Geometry: final body of the model. Coordinates: model frame, mm. A direction names the side the tool comes from. Give positions to 0.01 mm unless a question says otherwise; leave off trailing zeros. Write each loop counter-clockwise with the first axis right and the second up, starting at its lowest first coordinate (ties: lowest second). Pieces come first, ordered by that corner, then holes. Notation, with made-up numbers: M 67.25,31.25 L 119.25,31.25 A20 ccw 119.25,70.25 Z; hole C -39,55.25 d2. An arc over 180 degrees is marked long. One line per question, with ' | ' between items.
from build123d import *

# Parameters (mm, degrees)
BOX003_W               = 4.5
BOX003_H               = 5
BOX003_DEPTH           = 6
BOX003_PLACEMENT_ANGLE = 315
FILLET004_R            = 2.24
BOX002_W               = 19.2
BOX002_H               = 16.5
BOX002_DEPTH           = 6
FILLET005_R            = 2
BOX006_W               = 4.5
BOX006_H               = 5
BOX006_DEPTH           = 6
BOX006_PLACEMENT_ANGLE = 315
FILLET006_R            = 2.24
CYLINDER_R             = 9.75
CYLINDER_DEPTH         = 6
FILLET007_1_R          = 2
FILLET007_2_R          = 1


with BuildPart() as fillet004:
    # Box003 → Box003 (new body)
    with BuildSketch(Plane.XY):
        with Locations((2.25, 2.5)):
            Rectangle(BOX003_W, BOX003_H)
    extrude(amount=BOX003_DEPTH)


with BuildPart() as fillet004_1:
    # Box003 placement: moved
    add(fillet004.part.moved(Location((13.42, 28.5, 0))).rotate(Axis((13.42, 28.5, 0), (0, 0, 1)), BOX003_PLACEMENT_ANGLE))

    # Fillet004
    fillet004_edges = [fillet004_1.edges().sort_by_distance(p)[0] for p in [
        (16.955534, 32.035534, 3),
        (20.137514, 28.853553, 3),
    ]]
    fillet(fillet004_edges, radius=FILLET004_R)


with BuildPart() as fillet005:
    # Box002 → Box002 (new body)
    with BuildSketch(Plane.XY):
        with Locations((9.6, 8.25)):
            Rectangle(BOX002_W, BOX002_H)
    extrude(amount=BOX002_DEPTH)

    # Fillet005
    fillet005_edges = [fillet005.edges().sort_by_distance(p)[0] for p in [
        (0, 0, 3),
        (0, 16.5, 3),
        (19.2, 0, 3),
        (19.2, 16.5, 3),
    ]]
    fillet(fillet005_edges, radius=FILLET005_R)


with BuildPart() as fillet006:
    # Box006 → Box006 (new body)
    with BuildSketch(Plane.XY):
        with Locations((2.25, 2.5)):
            Rectangle(BOX006_W, BOX006_H)
    extrude(amount=BOX006_DEPTH)


with BuildPart() as fillet006_1:
    # Box006 placement: moved
    add(fillet006.part.moved(Location((2.6, 25.3, 0))).rotate(Axis((2.6, 25.3, 0), (0, 0, -1)), BOX006_PLACEMENT_ANGLE))

    # Fillet006
    fillet006_edges = [fillet006_1.edges().sort_by_distance(p)[0] for p in [
        (-0.935534, 28.835534, 3),
        (2.246447, 32.017514, 3),
    ]]
    fillet(fillet006_edges, radius=FILLET006_R)


with BuildPart() as fillet007:
    # Cylinder → Cylinder (new body)
    with BuildSketch(Plane(origin=(9.6, 21.3, 0), x_dir=(1, 0, 0), z_dir=(0, 0, 1))):
        Circle(CYLINDER_R)
    extrude(amount=CYLINDER_DEPTH)

    # Fusion025: union Fillet004, Fillet005, Fillet006
    add(fillet004_1.part)
    add(fillet005.part)
    add(fillet006_1.part)

    # Fillet007 1
    fillet007_1_edges = [fillet007.edges().sort_by_distance(p)[0] for p in [
        (4.596011, 29.66795, 3),
        (14.593947, 29.673947, 3),
        (17.822898, 26.538937, 3),
        (1.370866, 26.529134, 3),
    ]]
    fillet(fillet007_1_edges, radius=FILLET007_1_R)

    # Fillet007 2
    fillet007_2_edges = [fillet007.edges().sort_by_distance(p)[0] for p in [
        (1.207976, 16.336491, 3),
        (17.992024, 16.336491, 3),
    ]]
    fillet(fillet007_2_edges, radius=FILLET007_2_R)


solid = fillet007.part
(1) Draft query along Y for faces 6 (the face through (9, 15, 6)), 7 (the face through (17.025, 31.107, 3.042)), 8 (the face through (19.047, 15.268, 3.042)). Return one class per face: released by +Y, released by -Y, zero draft, split by the parting line, or undercut.
Working result:
face 6: zero draft | face 7: released by +Y | face 8: undercut
(2) First-contact query: P1, Ø8, axis at x = 11.5, y = 9, coming from the -Z side; P2, Ø2, axis at y = 27.5, z = 1, coming from the -X side; P3, Ø1.8, axis at y = 6.5, z = 2.5, coming from the +X side. Flat tips, straight axial feed; report the tip coordinate or a pass-through.
Working result:
P1: stops at z = 0 | P2: stops at x = 0.02 | P3: stops at x = 19.2
(3) Material intervals for L1, parallel to X at y = 7.5, z = 4; L2, parallel to Y at x = 15, z = 4; L3, parallel to Y at x = 8, z = 4.75, sorted ascending. Write a range as [from, to].
Working result:
L1: x = [0, 19.2] | L2: y = [0, 30.26] | L3: y = [0, 30.92]
(4) Cut plane A-A, the plane y = 10. Return loops of the section in (x, z), then the cut area to 3 significant figures.
Working result:
outline: M 0,0 L 19.2,0 L 19.2,6 L 0,6 Z | area: 115 mm^2
(5) Set-up query: faces 1 (the face through (9.65, 31.05, 2.96)), 2 (the face through (0.153, 15.268, 3.042)), 3 (the face through (9, 16, 0)), 4 (the face through (19.2, 8, 3)), 5 (the face through (0, 8, 3)). Return all of +Z, -Z, +X, -X, +Y, -Y with unobstructed straight access to the full face (end or side cutting, diameter ignored); none if empty.
Working result:
face 1: +Z, -Z, +Y | face 2: +Z, -Z, -X | face 3: -Z, +X, -X, +Y, -Y | face 4: +Z, -Z, +X, -Y | face 5: +Z, -Z, -X, -Y
